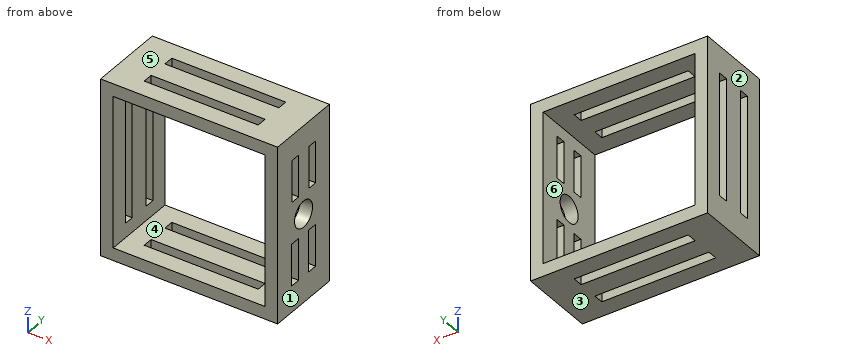
from build123d import *

# Parameters (mm, degrees)
SKETCH2_W           = 35
SKETCH2_H           = 35
BOSS_EXTRUDE1_DEPTH = 10
SKETCH3_W           = 35
SKETCH3_H           = 35
SKETCH3_W_2         = 30
SKETCH3_H_2         = 30
BOSS_EXTRUDE2_DEPTH = 15
SKETCH4_W           = 35
SKETCH4_H           = 35
BOSS_EXTRUDE3_DEPTH = 15
CUT_EXTRUDE1_START  = -40
SKETCH5_R           = 3.05
CUT_EXTRUDE1_DEPTH  = 40
SKETCH6_R           = 2.6
SKETCH6_W           = 8.296096318
SKETCH6_H           = 2.00000001
SKETCH6_H_2         = 2.000000011
CUT_EXTRUDE2_DEPTH  = 2.5
CUT_EXTRUDE3_REACH  = 48.435
SKETCH7_W           = 22.518110106
SKETCH7_H           = 2
SKETCH8_W           = 24.260657828
SKETCH8_H           = 2
CUT_EXTRUDE4_DEPTH  = 2.5


with BuildPart() as part:
    # Sketch2 → Boss-Extrude1 (new body)
    with BuildSketch(Plane(origin=(0, 0, 0), x_dir=(1, 0, 0), z_dir=(0, 1, 0))):
        Rectangle(SKETCH2_W, SKETCH2_H)
    extrude(amount=BOSS_EXTRUDE1_DEPTH)


with BuildPart() as body_2:
    # Sketch3 → Boss-Extrude2 (new body)
    with BuildSketch(Plane(origin=(0, 10, 0), x_dir=(1, 0, 0), z_dir=(0, 1, 0))):
        Rectangle(SKETCH3_W, SKETCH3_H)
        Rectangle(SKETCH3_W_2, SKETCH3_H_2, mode=Mode.SUBTRACT)
    extrude(amount=BOSS_EXTRUDE2_DEPTH)

    # Sketch6 → Cut-Extrude2 (cut)
    with BuildSketch(Plane(origin=(17.5, 0, 0), x_dir=(0, 0, -1), z_dir=(1, 0, 0))):
        with Locations((0, 17.5)):
            Circle(SKETCH6_R)
        with Locations((8.1389247, 15.064547851)):
            Rectangle(SKETCH6_W, SKETCH6_H)
        with Locations((8.1389247, 20.000000005)):
            Rectangle(SKETCH6_W, SKETCH6_H)
        with Locations((-8.361055595, 15.090047995)):
            Rectangle(SKETCH6_W, SKETCH6_H)
        with Locations((-8.361055595, 20.025500149)):
            Rectangle(SKETCH6_W, SKETCH6_H_2)
    extrude(amount=-CUT_EXTRUDE2_DEPTH, mode=Mode.SUBTRACT)

    # Cut-Extrude3: up to this face of the body (flat: up to its plane)
    cut_extrude3_end = Plane(body_2.part.faces().sort_by_distance((0, 17.5, -17.5))[0])
    # Sketch7 → Cut-Extrude3 (cut, up to the picked face)
    with BuildSketch(Plane.XY.offset(17.5), mode=Mode.PRIVATE) as cut_extrude3_sk1:
        with Locations((0, 20.5)):
            Rectangle(SKETCH7_W, SKETCH7_H)
    cut_extrude3_tool1 = split(extrude(cut_extrude3_sk1.sketch, amount=-CUT_EXTRUDE3_REACH, mode=Mode.PRIVATE), bisect_by=cut_extrude3_end, keep=Keep.BOTH, mode=Mode.PRIVATE)
    # Sketch7 → Cut-Extrude3 (cut, up to the picked face)
    with BuildSketch(Plane.XY.offset(17.5), mode=Mode.PRIVATE) as cut_extrude3_sk2:
        with Locations((0, 14.5)):
            Rectangle(SKETCH7_W, SKETCH7_H)
    cut_extrude3_tool2 = split(extrude(cut_extrude3_sk2.sketch, amount=-CUT_EXTRUDE3_REACH, mode=Mode.PRIVATE), bisect_by=cut_extrude3_end, keep=Keep.BOTH, mode=Mode.PRIVATE)
    add(cut_extrude3_tool1.solids().sort_by(Axis((0, 20.5, 17.5), (0, 0, -1)))[0], mode=Mode.SUBTRACT)
    add(cut_extrude3_tool2.solids().sort_by(Axis((0, 14.5, 17.5), (0, 0, -1)))[0], mode=Mode.SUBTRACT)

    # Sketch8 → Cut-Extrude4 (cut)
    with BuildSketch(Plane.ZY.offset(17.5)):
        with Locations((0, 20.5)):
            Rectangle(SKETCH8_W, SKETCH8_H)
        with Locations((0, 14.5)):
            Rectangle(SKETCH8_W, SKETCH8_H)
    extrude(amount=-CUT_EXTRUDE4_DEPTH, mode=Mode.SUBTRACT)


with BuildPart() as body_3:
    # Sketch4 → Boss-Extrude3 (new body)
    with BuildSketch(Plane(origin=(0, 25, 0), x_dir=(1, 0, 0), z_dir=(0, 1, 0))):
        Rectangle(SKETCH4_W, SKETCH4_H)
    extrude(amount=BOSS_EXTRUDE3_DEPTH)


with BuildPart() as cut_extrude1_tool:
    # Sketch5 → Cut-Extrude1 (new body)
    with BuildSketch(Plane(origin=(0, 40, 0), x_dir=(1, 0, 0), z_dir=(0, 1, 0)).offset(CUT_EXTRUDE1_START)):
        with Locations(Location((0, 0, 0), (0, 0, 270))):
            Circle(SKETCH5_R)
    extrude(amount=CUT_EXTRUDE1_DEPTH)


with BuildPart() as part_1:
    add(part.part)

    # Cut-Extrude1: cut by cut_extrude1_tool
    add(cut_extrude1_tool.part, mode=Mode.SUBTRACT)


with BuildPart() as body_3_1:
    add(body_3.part)

    # Cut-Extrude1: cut by cut_extrude1_tool
    add(cut_extrude1_tool.part, mode=Mode.SUBTRACT)


solid = body_2.part
Work out the finished part from the listing and answer in its coordinate system (mm). Face numbers are marked on the shaded views. A direction names the side the tool comes from. Coordinates: 2 decimals unless noted, no trailing zeros. Order: outer loops, then holes, each group sorted by start corner. A loop starts at its lowest first (then second) coordinate and runs counter-clockwise, first axis right, second up. Notation, with made-up numbers: (-3.5, -31) - (3.5, -31) arc R12 cw to (3.5, -11) - close; hole circle Ø5 at (46, 68). An arc over 180 degrees is marked (long way). Put each result on its own line as item: value. Start each with the question number.
1) For a pull along X with two mould halves and no side action, classify the marked faces 1, 2, 3 and 4 as released by +X, released by -X, zero draft, split by the parting line, or undercut.
2) Find section A-A (x = -8). Give the vertices of the cut face in (y, z), plus the area to 3 significant figures.
3) Find section B-B (z = -13). Give the vertices of the cut face in (x, y), plus the area to 3 significant figures.
4) Find the intervals of material crossed by line 1 (X direction, y = 23, z = 7.5); line 2 (Y direction, x = 16, z = 0), in increasing order. Write a range as from..to.
5) For the marked faces 5 and 6, determine the directions among +Z, -Z, +X, -X, +Y, -Y from which every point of the face is accessible in a straight line to the end or side of a thin tool.
6) Find section C-C (y = 11.25). Give the vertices of the cut face in (x, z), plus the area to 3 significant figures.
7) Find section D-D (z = 0). Give the vertices of the cut face in (x, y).
Results list:
1. face 1: released by +X
1. face 2: released by -X
1. face 3: zero draft
1. face 4: undercut
2. outline: (10, -17.5) - (13.5, -17.5) - (13.5, -15) - (10, -15) - close; (10, 15) - (13.5, 15) - (13.5, 17.5) - (10, 17.5) - close; (15.5, -17.5) - (19.5, -17.5) - (19.5, -15) - (15.5, -15) - close; (15.5, 15) - (19.5, 15) - (19.5, 17.5) - (15.5, 17.5) - close; (21.5, -17.5) - (25, -17.5) - (25, -15) - (21.5, -15) - close; (21.5, 15) - (25, 15) - (25, 17.5) - (21.5, 17.5) - close
2. area: 55.0 mm^2
3. outline: (-17.5, 10) - (-15, 10) - (-15, 25) - (-17.5, 25) - close; (15, 10) - (17.5, 10) - (17.5, 25) - (15, 25) - close
3. area: 75.0 mm^2
4. line 1: x = -17.5..-15, 15..17.5
4. line 2: y = 10..14.9, 20.1..25
5. face 5: +Z, +X, -X, +Y, -Y
5. face 6: +Y, -Y
6. outline: (-17.5, -17.5) - (17.5, -17.5) - (17.5, 17.5) - (-17.5, 17.5) - close; hole (-15, -15) - (15, -15) - (15, 15) - (-15, 15) - close
6. area: 325 mm^2
7. outline: (-17.5, 10) - (-15, 10) - (-15, 13.5) - (-17.5, 13.5) - close; (-17.5, 15.5) - (-15, 15.5) - (-15, 19.5) - (-17.5, 19.5) - close; (-17.5, 21.5) - (-15, 21.5) - (-15, 25) - (-17.5, 25) - close; (15, 10) - (17.5, 10) - (17.5, 14.9) - (15, 14.9) - close; (15, 20.1) - (17.5, 20.1) - (17.5, 25) - (15, 25) - close
